Part print with two shaded views. Sizes in mm from the minimum x, y, z corner. A direction names the side the tool comes from. Round coordinates to 2 decimals unless told otherwise and drop trailing zeros. Loops run counter-clockwise (first coordinate to the right, second up) from the corner with the lowest first, then second, coordinate; pieces in that order, holes last. Notation, with made-up numbers: M -24,-10 L -4,-10 A11 ccw -4,5 Z; hole C 75.25,-28 d1. An arc over 180 degrees is marked long. Use a Markdown table: item, result. Add a question column.
Item 1: Wall check: L1, parallel to Y at x = 1, z = 2; L2, parallel to X at y = 14.5, z = 3.5; L3, parallel to Z at x = 2.25, y = 24. Give the ranges that are in metal, low to high. Write a range as from..to.
Item 2: Saw through at A-A on x = 3.5. Write the cut outline in (y, z).
Item 3: Saw through at C-C on y = 13.25. Write the cut outline in (x, z), then the cut area to 3 significant figures.
Item 4: Tool access for the marked faces 1 and 2: list every direction of +Z, -Z, +X, -X, +Y, -Y with a clear straight run to the whole face (end or side of a thin tool).
Item 5: Saw through at B-B on z = 3.5. Write the cut outline in (x, y).
Item 6: Saw through at D-D on y = 2.5. Write the cut outline in (x, z).
Item 7: Pin check, flat tips, straight feed: P1, Ø1.5, axis at y = 17.5, z = 2, coming from the +X side; P2, Ø1, axis at x = 5.5, y = 4.5, coming from the -Z side (3 decimals); P3, Ø1.5, axis at x = 1.5, y = 14.5, coming from the +Z side. Stop position of each tip, or through.
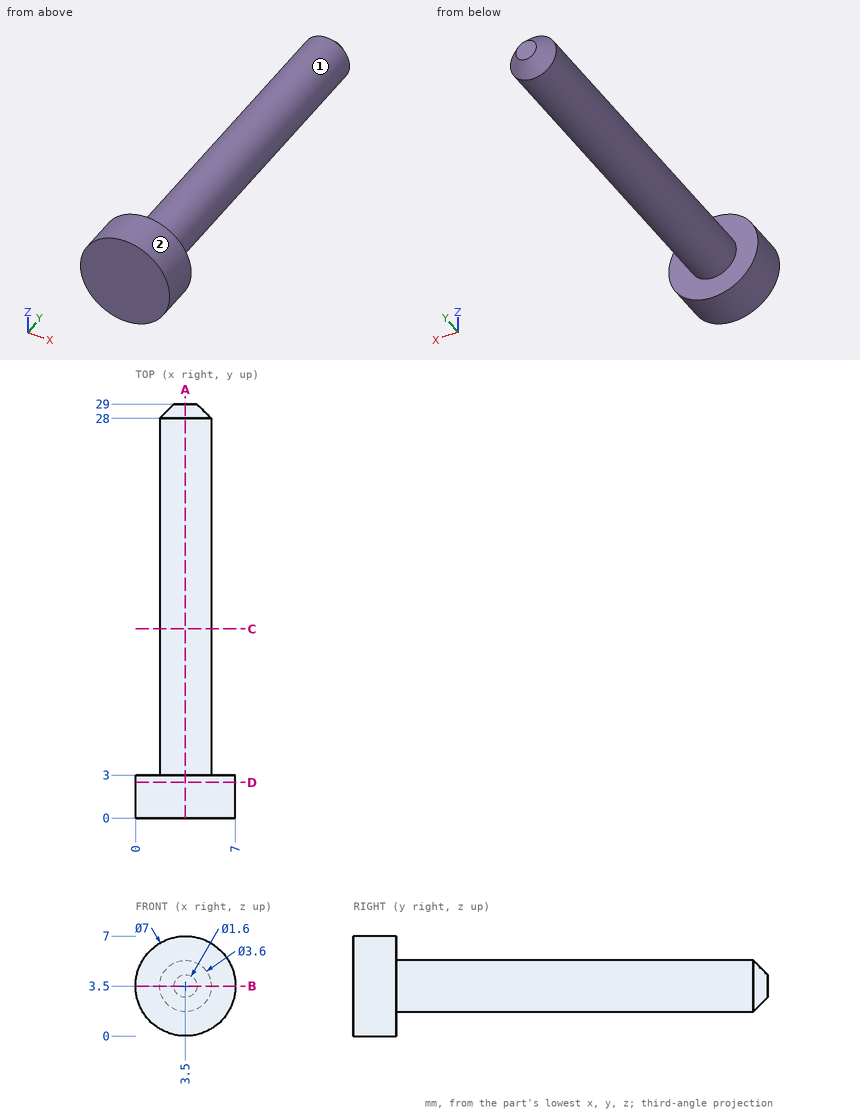
Entries:
| question | item | result |
|---|---|---|
| 1 | L1 | 0..3 |
| 1 | L2 | 1.7..5.3 |
| 1 | L3 | 2.2..4.8 |
| 2 | outline | M 0,0 L 3,0 L 3,1.7 L 28,1.7 L 29,2.7 L 29,4.3 L 28,5.3 L 3,5.3 L 3,7 L 0,7 Z |
| 3 | outline | C 3.5,3.5 d3.6 |
| 3 | area | 10.2 mm2 |
| 4 | face 1 | +Y |
| 4 | face 2 | +Y, -Y |
| 5 | outline | M 0,0 L 7,0 L 7,3 L 5.3,3 L 5.3,28 L 4.3,29 L 2.7,29 L 1.7,28 L 1.7,3 L 0,3 Z |
| 6 | outline | C 3.5,3.5 d7 |
| 7 | P1 | x = 5.14 |
| 7 | P2 | z = 2.505 |
| 7 | P3 | z = 4.8 |
